```python
from build123d import *

# Parameters (mm, degrees)
SKETCH1_R           = 18.5
SKETCH1_R_2         = 6.25
SKETCH1_R_3         = 1.6
SKETCH1_R_4         = 2.1
BOSS_EXTRUDE1_DEPTH = 6
BOSS_EXTRUDE2_START = -6
SKETCH3_R           = 2
BOSS_EXTRUDE2_DEPTH = 11.395208
SKETCH4_R           = 3.5
CUT_EXTRUDE1_DEPTH  = 5


with BuildPart() as part:
    # Sketch1 → Boss-Extrude1 (new body)
    with BuildSketch(Plane.XY):
        with Locations(Location((0, 0, 0), (0, 0, 180))):
            Circle(SKETCH1_R)
        with Locations(Location((0, 7, 0), (0, 0, 180))):
            Circle(SKETCH1_R_2, mode=Mode.SUBTRACT)
        with Locations(Location((15.5, 0, 0), (0, 0, 180))):
            Circle(SKETCH1_R_3, mode=Mode.SUBTRACT)
        with Locations(Location((7.75, -13.423393759, 0), (0, 0, 180))):
            Circle(SKETCH1_R_3, mode=Mode.SUBTRACT)
        with Locations(Location((-7.75, -13.423393759, 0), (0, 0, 180))):
            Circle(SKETCH1_R_3, mode=Mode.SUBTRACT)
        with Locations(Location((-15.5, 0, 0), (0, 0, 180))):
            Circle(SKETCH1_R_3, mode=Mode.SUBTRACT)
        with Locations(Location((-7.75, 13.423393759, 0), (0, 0, 180))):
            Circle(SKETCH1_R_3, mode=Mode.SUBTRACT)
        with Locations(Location((7.75, 13.423393759, 0), (0, 0, 180))):
            Circle(SKETCH1_R_3, mode=Mode.SUBTRACT)
        with Locations(Location((13.423393759, 7.75, 0), (0, 0, 180))):
            Circle(SKETCH1_R_4, mode=Mode.SUBTRACT)
        with Locations(Location((0, -15.5, 0), (0, 0, 180))):
            Circle(SKETCH1_R_4, mode=Mode.SUBTRACT)
        with Locations(Location((-13.423393759, 7.75, 0), (0, 0, 180))):
            Circle(SKETCH1_R_4, mode=Mode.SUBTRACT)
    extrude(amount=BOSS_EXTRUDE1_DEPTH)

    # Sketch3 → Boss-Extrude2 (add)
    with BuildSketch(Plane.XY.offset(6).offset(BOSS_EXTRUDE2_START)):
        with BuildLine():
            ThreePointArc((18.5, 0), (0, -18.5), (-18.5, 0))
            Line((-18.5, 0), (-18.5, -31.300991))
            Line((-18.5, -31.300991), (18.5, -31.300991))
            Line((18.5, -31.300991), (18.5, 0))
        make_face()
        with Locations(Location((-13.5, -21.300991, 0), (0, 0, 270))):
            Circle(SKETCH3_R, mode=Mode.SUBTRACT)
        with Locations(Location((13.5, -21.300991, 0), (0, 0, 270))):
            Circle(SKETCH3_R, mode=Mode.SUBTRACT)
    extrude(amount=BOSS_EXTRUDE2_DEPTH)

    # Sketch4 → Cut-Extrude1 (cut)
    with BuildSketch(Plane(origin=(0, 0, 0), x_dir=(-1, 0, 0), z_dir=(0, 0, -1))):
        with Locations((-13.5, -21.300991)):
            Circle(SKETCH4_R)
        with Locations((13.5, -21.300991)):
            Circle(SKETCH4_R)
    extrude(amount=-CUT_EXTRUDE1_DEPTH, mode=Mode.SUBTRACT)


solid = part.part
```
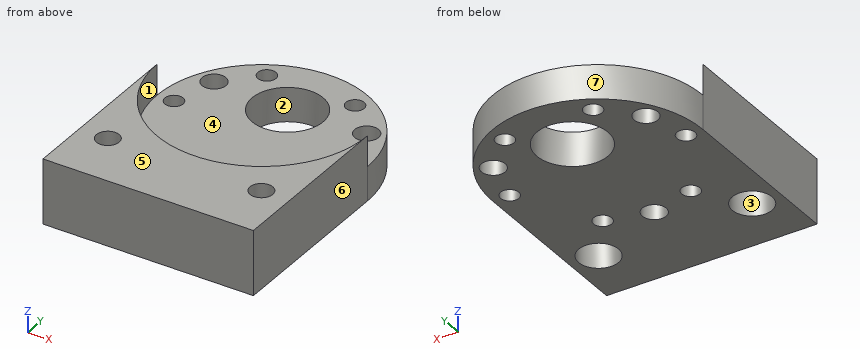
Model file for the job. Use its own axes, mm. Face numbers are marked on the shaded views. A direction names the side the tool comes from. Give positions to 0.01 mm unless a question says otherwise; leave off trailing zeros. Write each loop counter-clockwise with the first axis right and the second up, starting at its lowest first coordinate (ties: lowest second). Pieces come first, ordered by that corner, then holes. Notation, with made-up numbers: M 70.5,34.5 L 85.5,34.5 A23 ccw 85.5,46.5 Z; hole C 63,39.25 d11. An arc over 180 degrees is marked long. Use a Markdown table: item, result.
1) Cut at A-A (x = 0). List the corners of the cut face in (y, z).
Responses:
| item | result |
|---|---|
| outline | M -31.3,0 L -17.6,0 L -17.6,6 L -18.5,6 L -18.5,11.4 L -31.3,11.4 Z; M -13.4,0 L 0.75,0 L 0.75,6 L -13.4,6 Z; M 13.25,0 L 18.5,0 L 18.5,6 L 13.25,6 Z |
2) Cut at B-B (y = 7). List the corners of the cut face in (x, z), and give its area (3 significant figures).
Responses:
| item | result |
|---|---|
| outline | M -17.12,0 L -15.38,0 L -15.38,6 L -17.12,6 Z; M -11.46,0 L -6.25,0 L -6.25,6 L -11.46,6 Z; M 6.25,0 L 11.46,0 L 11.46,6 L 6.25,6 Z; M 15.38,0 L 17.12,0 L 17.12,6 L 15.38,6 Z |
| area | 83.4 mm2 |
3) Drill centre lines: line 1 (X direction, y = 7.75, z = 2.2); line 2 (X direction, y = 12, z = 1.75); line 3 (Y direction, x = -7.75, z = 2.4). Where is each one in solid material? Low to high. Write a range as from..to.
Responses:
| item | result |
|---|---|
| line 1 | x = -16.8..-15.52, -11.32..-6.2, 6.2..11.32, 15.52..16.8 |
| line 2 | x = -14.08..-8.48, -7.02..-3.75, 3.75..7.02, 8.48..14.08 |
| line 3 | y = -31.3..-15.02, -11.82..11.82, 15.02..16.8 |
4) Tool access for the marked faces 1, 2 and 3: list every direction of +Z, -Z, +X, -X, +Y, -Y with a clear straight run to the whole face (end or side of a thin tool).
Responses:
| item | result |
|---|---|
| face 1 | +Z, +Y |
| face 2 | +Z, -Z |
| face 3 | -Z |
5) Cut at C-C (z = 10.75). List the corners of the cut face in (x, y).
Responses:
| item | result |
|---|---|
| outline | M -18.5,-31.3 L 18.5,-31.3 L 18.5,0 A18.5 cw -18.5,0 Z; hole C -13.5,-21.3 d4; hole C 13.5,-21.3 d4 |
6) Pull direction X, two halves, no side cores. Call the marked faces 4, 5, 6 and 7: +X half, -X half, draft (parallel to the pull), parting line (faces both ways), or undercut.
Responses:
| item | result |
|---|---|
| face 4 | undercut |
| face 5 | draft |
| face 6 | +X half |
| face 7 | parting line |
7) Cut at D-D (y = -1). Give the number of separate pieces and of enclosed holes in the cut face, and give its area (3 significant figures).
Responses:
| item | result |
|---|---|
| separate pieces | 3 |
| enclosed holes | 0 |
| area | 192 mm2 |
8) Pin check, flat tips, straight feed: pin 1 (4 mm diameter, centred on x = 15.5, y = 0, fed in from -Z); pin 2 (4 mm diameter, centred on x = -13.42, y = 7.75, fed in from -Z); pin 3 (4 mm diameter, centred on x = -7.75, y = 13.42, fed in from +Z). Stop position of each tip, or through.
Responses:
| item | result |
|---|---|
| pin 1 | stops at z = 0 |
| pin 2 | passes through |
| pin 3 | stops at z = 6 |
